from build123d import *

# Parameters (mm, degrees)
EXTRUDE002_DEPTH = 10
EXTRUDE003_DEPTH = 10
EXTRUDE004_DEPTH = 10
EXTRUDE005_DEPTH = 10
CIRCLE001_R      = 2.096161
EXTRUDE001_DEPTH = 10
EXTRUDE_DEPTH    = 10


with BuildPart() as extrude002:
    # DWire008 → Extrude002 (new body)
    with BuildSketch(Plane.XY):
        Polygon((-6.57, -8.2), (-7.031056, -8.2), (-8.2, -8.2), (-8.2, -7.031056), (-8.2, -6.57), (-7.66, -6.57), (-6.57, -7.66), align=None)
    extrude(amount=EXTRUDE002_DEPTH)


with BuildPart() as extrude003:
    # DWire009 → Extrude003 (new body)
    with BuildSketch(Plane.XY):
        Polygon((8.2, 7.031056), (8.2, 8.2), (7.031056, 8.2), (6.57, 8.2), (6.57, 7.66), (7.66, 6.57), (8.2, 6.57), align=None)
    extrude(amount=EXTRUDE003_DEPTH)


with BuildPart() as extrude004:
    # DWire010 → Extrude004 (new body)
    with BuildSketch(Plane.XY):
        Polygon((8.2, -6.57), (8.2, -7.031056), (8.2, -8.2), (7.031056, -8.2), (6.57, -8.2), (6.57, -7.66), (7.66, -6.57), align=None)
    extrude(amount=EXTRUDE004_DEPTH)


with BuildPart() as extrude005:
    # DWire011 → Extrude005 (new body)
    with BuildSketch(Plane.XY):
        Polygon((-8.2, 6.57), (-8.2, 7.031056), (-8.2, 8.2), (-7.031056, 8.2), (-6.57, 8.2), (-6.57, 7.66), (-7.66, 6.57), align=None)
    extrude(amount=EXTRUDE005_DEPTH)


with BuildPart() as extrude001:
    # Circle001 → Extrude001 (new body)
    with BuildSketch(Plane.XY):
        Circle(CIRCLE001_R)
    extrude(amount=EXTRUDE001_DEPTH)


with BuildPart() as v_slot_20x20:
    # Sketch001 → Extrude (new body)
    with BuildSketch(Plane(origin=(0, 0, 0), x_dir=(0, 1, 0), z_dir=(0, 0, 1))):
        with BuildLine():
            ThreePointArc((10, 8.5), (9.56066, 9.56066), (8.5, 10))
            Line((8.5, 10), (4.5, 10))
            Line((4.5, 10), (2.89, 8.315116))
            Line((2.89, 8.315116), (2.89, 8.2))
            Line((2.89, 8.2), (5.5, 8.2))
            Line((5.5, 8.2), (5.5, 6.56))
            Line((5.5, 6.56), (2.84, 3.9))
            Line((2.84, 3.9), (0.21, 3.9))
            Line((0.21, 3.9), (0, 3.69))
            Line((0, 3.69), (-0.21, 3.9))
            Line((-0.21, 3.9), (-2.84, 3.9))
            Line((-2.84, 3.9), (-5.5, 6.56))
            Line((-5.5, 6.56), (-5.5, 8.2))
            Line((-5.5, 8.2), (-2.89, 8.2))
            Line((-2.89, 8.2), (-2.89, 8.315116))
            Line((-2.89, 8.315116), (-4.5, 10))
            Line((-4.5, 10), (-8.5, 10))
            ThreePointArc((-8.5, 10), (-9.56066, 9.56066), (-10, 8.5))
            Line((-10, 8.5), (-10, 4.5))
            Line((-10, 4.5), (-8.315116, 2.89))
            Line((-8.315116, 2.89), (-8.2, 2.89))
            Line((-8.2, 2.89), (-8.2, 5.5))
            Line((-8.2, 5.5), (-6.56, 5.5))
            Line((-6.56, 5.5), (-3.9, 2.84))
            Line((-3.9, 2.84), (-3.9, 0.21))
            Line((-3.9, 0.21), (-3.69, 0))
            Line((-3.69, 0), (-3.9, -0.21))
            Line((-3.9, -0.21), (-3.9, -2.84))
            Line((-3.9, -2.84), (-6.56, -5.5))
            Line((-6.56, -5.5), (-8.2, -5.5))
            Line((-8.2, -5.5), (-8.2, -2.89))
            Line((-8.2, -2.89), (-8.315116, -2.89))
            Line((-8.315116, -2.89), (-10, -4.5))
            Line((-10, -4.5), (-10, -8.5))
            ThreePointArc((-10, -8.5), (-9.56066, -9.56066), (-8.5, -10))
            Line((-8.5, -10), (-4.5, -10))
            Line((-4.5, -10), (-2.89, -8.315116))
            Line((-2.89, -8.315116), (-2.89, -8.2))
            Line((-2.89, -8.2), (-5.5, -8.2))
            Line((-5.5, -8.2), (-5.5, -6.56))
            Line((-5.5, -6.56), (-2.84, -3.9))
            Line((-2.84, -3.9), (-0.21, -3.9))
            Line((-0.21, -3.9), (0, -3.69))
            Line((0, -3.69), (0.21, -3.9))
            Line((0.21, -3.9), (2.84, -3.9))
            Line((2.84, -3.9), (5.5, -6.56))
            Line((5.5, -6.56), (5.5, -8.2))
            Line((5.5, -8.2), (2.89, -8.2))
            Line((2.89, -8.2), (2.89, -8.315116))
            Line((2.89, -8.315116), (4.5, -10))
            Line((4.5, -10), (8.5, -10))
            ThreePointArc((8.5, -10), (9.56066, -9.56066), (10, -8.5))
            Line((10, -8.5), (10, -4.5))
            Line((10, -4.5), (8.315116, -2.89))
            Line((8.315116, -2.89), (8.2, -2.89))
            Line((8.2, -2.89), (8.2, -5.5))
            Line((8.2, -5.5), (6.56, -5.5))
            Line((6.56, -5.5), (3.9, -2.84))
            Line((3.9, -2.84), (3.9, -0.21))
            Line((3.9, -0.21), (3.69, 0))
            Line((3.69, 0), (3.9, 0.21))
            Line((3.9, 0.21), (3.9, 2.84))
            Line((3.9, 2.84), (6.56, 5.5))
            Line((6.56, 5.5), (8.2, 5.5))
            Line((8.2, 5.5), (8.2, 2.89))
            Line((8.2, 2.89), (8.315116, 2.89))
            Line((8.315116, 2.89), (10, 4.5))
            Line((10, 4.5), (10, 8.5))
        make_face()
    extrude(amount=EXTRUDE_DEPTH)

    # Cut: cut Extrude001
    add(extrude001.part, mode=Mode.SUBTRACT)

    # Cut001: cut Extrude005
    add(extrude005.part, mode=Mode.SUBTRACT)

    # Cut002: cut Extrude004
    add(extrude004.part, mode=Mode.SUBTRACT)

    # Cut003: cut Extrude003
    add(extrude003.part, mode=Mode.SUBTRACT)

    # Cut004: cut Extrude002
    add(extrude002.part, mode=Mode.SUBTRACT)


solid = v_slot_20x20.part
Part model, mm, in its own coordinate system. A direction names the side the tool comes from. Coordinates: 2 decimals unless noted, no trailing zeros. Write each loop counter-clockwise with the first axis right and the second up, starting at its lowest first coordinate (ties: lowest second). Pieces come first, ordered by that corner, then holes. Notation, with made-up numbers: M -6.75,68 L -0.75,68 A22 ccw -0.75,98 Z; hole C 6,-32 d5. An arc over 180 degrees is marked long. Return JSON: item names as keys, results as strings.
1. Saw through at D-D, the plane z = 6. Count the separate pieces of the cut face and the enclosed holes in it, then the cut area to 3 significant figures.
Determined:
{"separate pieces": "1", "enclosed holes": "5", "area": "162 mm²"}
2. Saw through at C-C, the plane x = 0.75. Write the cut outline in (y, z), then the cut area to 3 significant figures.
Determined:
{"outline": "M -3.9,0 L -1.96,0 L -1.96,10 L -3.9,10 Z; M 1.96,0 L 3.9,0 L 3.9,10 L 1.96,10 Z", "area": "38.9 mm²"}
3. Flat gauge pins, fed straight in: pin 1 Ø4 at (x, z) = (0.5, 3.5) entering from -Y; pin 2 Ø2 at (x, z) = (-3, 6.5) entering from -Y; pin 3 Ø6 at (x, y) = (-4, 3) entering from -Z; pin 4 Ø3 at (y, z) = (-1.5, 6.5) entering from -X. Where does each tip first touch, or does it go through?
Determined:
{"pin 1": "y = -3.9", "pin 2": "y = -9.48", "pin 3": "z = 0", "pin 4": "x = -8.43"}
4. Saw through at A-A, the plane y = 6.25. Write the cut outline in (x, z), then the cut area to 3 significant figures.
Determined:
{"outline": "M -10,0 L -5.19,0 L -5.19,10 L -10,10 Z; M 5.19,0 L 10,0 L 10,10 L 5.19,10 Z", "area": "96.2 mm²"}
5. Pull direction X, two halves, no side cores. Call faces 1 (the face through (-7, 5.5, 5)), 2 (the face through (-7, -10, 5)), 3 (the face through (-3.9, 2, 5)): pulls with the +X half, pulls with the -X half, needs draft (parallel to the pull), parting line crosses it, or undercut.
Determined:
{"face 1": "undercut", "face 2": "needs draft", "face 3": "pulls with the -X half"}
6. Probe L1, parallel to X at y = -4, z = 8.75; L2, parallel to X at y = -3.5, z = 5.75. List the from-to ranges inside material, lowest first.
Determined:
{"L1": "-9.48 to -8.2, -5.06 to -2.94, 2.94 to 5.06, 8.2 to 9.48", "L2": "-8.95 to -8.2, -4.56 to 4.56, 8.2 to 8.95"}
7. Saw through at B-B, the plane x = -7. Write the cut outline in (y, z).
Determined:
{"outline": "M -10,0 L -8.2,0 L -8.2,10 L -10,10 Z; M -7.23,0 L -5.5,0 L -5.5,10 L -7.23,10 Z; M 5.5,0 L 7.23,0 L 7.23,10 L 5.5,10 Z; M 8.2,0 L 10,0 L 10,10 L 8.2,10 Z"}
8. 3-axis set-ups, long thin cutter, end or side, ignore diameter. For faces 4 (the face through (-2, 3.9, 5)), 5 (the face through (5.5, -7, 5)), 6 (the face through (10, 6, 5)), 7 (the face through (3.9, -2, 5)), 8 (the face through (7, 10, 5)): which of +Z, -Z, +X, -X, +Y, -Y reach the whole face in a straight line?
Determined:
{"face 4": "+Z, -Z, +Y", "face 5": "+Z, -Z", "face 6": "+Z, -Z, +X, +Y, -Y", "face 7": "+Z, -Z, +X", "face 8": "+Z, -Z, +X, -X, +Y"}
